from build123d import *

# Parameters (mm, degrees)
SKETCH1_R           = 12.8
BOSS_EXTRUDE1_DEPTH = 100
SKETCH3_R           = 8.348764046
BOSS_EXTRUDE3_DEPTH = 10
CHAMFER3_SIZE       = 8
CHAMFER4_SIZE       = 8


with BuildPart() as part:
    # Sketch1 → Boss-Extrude1 (new body)
    with BuildSketch(Plane(origin=(0, 0, 0), x_dir=(1, 0, 0), z_dir=(0, 1, 0))):
        with Locations(Location((0, 0, 0), (0, 0, 270))):
            Circle(SKETCH1_R)
    extrude(amount=BOSS_EXTRUDE1_DEPTH)

    # Sketch3 → Boss-Extrude3 (add)
    with BuildSketch(Plane(origin=(0, 100, 0), x_dir=(1, 0, 0), z_dir=(0, 1, 0))):
        with Locations(Location((0, 0, 0), (0, 0, 270))):
            Circle(SKETCH3_R)
    extrude(amount=BOSS_EXTRUDE3_DEPTH)

    # Chamfer3
    chamfer3_edges = [part.edges().sort_by_distance(p)[0] for p in [
        (0, 110, -8.348764046),
    ]]
    chamfer(chamfer3_edges, length=CHAMFER3_SIZE)

    # Chamfer4
    # the kernel refuses this chamfer: 8 mm, written as the material it takes off along each edge
    with BuildSketch(Plane(origin=(0, 100, 0), x_dir=(0, 0, 1), z_dir=(-1, 0, 0))) as chamfer4_piece_1_section:
        Polygon((12.8 - CHAMFER4_SIZE, 0), (12.8, -CHAMFER4_SIZE), (12.8, 0), align=None)
    chamfer4_piece_1 = revolve(axis=Axis((0, 100, 0), (0, 1, 0)), mode=Mode.PRIVATE)
    chamfer4_piece_1 = chamfer4_piece_1 - Plane(origin=(0, 94.200473473, 0), x_dir=(0, 0, 1), z_dir=(0, -1, 0)) * Cylinder(8.348764046, 52, mode=Mode.PRIVATE)
    add(chamfer4_piece_1, mode=Mode.SUBTRACT)


solid = part.part
Part model, mm, in its own coordinate system. Coordinates: 2 decimals unless noted, no trailing zeros. Order: outer loops, then holes, each group sorted by start corner. A loop starts at its lowest first (then second) coordinate and runs counter-clockwise, first axis right, second up. Notation, with made-up numbers: M 76.5,64 L 83.5,64 A11 cw 83.5,78 Z; hole C 79,72.25 d6. An arc over 180 degrees is marked long. Use a Markdown table: item, result.
(1) Cut at A-A on y = 23. Write the cut outline in (x, z), then the cut area to 3 significant figures.
A:
| item | result |
|---|---|
| outline | C 0,0 d25.6 |
| area | 515 mm^2 |
(2) Flat gauge pins, fed straight in: pin 1 (1 mm diameter, centred on x = -1.5, y = 23, fed in from +Z); pin 2 (1.5 mm diameter, centred on y = 69, z = 9, fed in from +X); pin 3 (1 mm diameter, centred on x = 7, z = -2, fed in from +Y). Where does each tip first touch, or does it go through?
A:
| item | result |
|---|---|
| pin 1 | stops at z = 12.76 |
| pin 2 | stops at x = 9.79 |
| pin 3 | stops at y = 103.57 |
(3) Probe L1, parallel to X at y = 97.5, z = -4.5; L2, parallel to Z at x = 11.5, y = 11.5; L3, parallel to Y at x = -1, z = -11.5. List the from-to ranges inside material, lowest first.
A:
| item | result |
|---|---|
| L1 | x = -7.03 to 7.03 |
| L2 | z = -5.62 to 5.62 |
| L3 | y = 0 to 93.26 |
